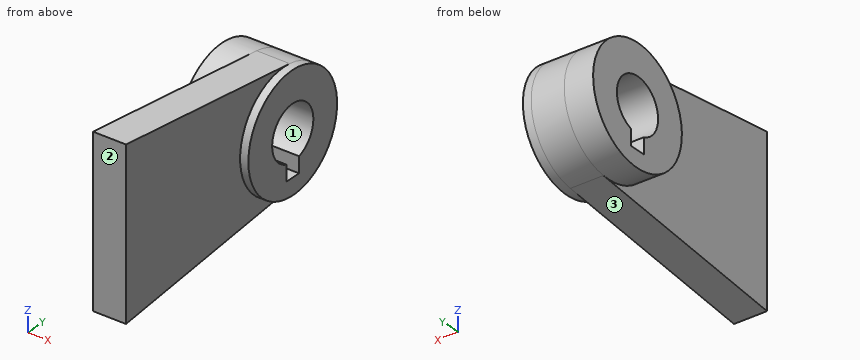
from build123d import *
from build123d.topology import SkipClean

# Parameters (mm, degrees)
SALIENTE_EXTRUIR3_DEPTH = 16
CROQUIS6_R              = 28
SALIENTE_EXTRUIR4_DEPTH = 4
SALIENTE_EXTRUIR5_START = 14
CROQUIS7_R              = 28
SALIENTE_EXTRUIR5_DEPTH = 14
CORTAR_EXTRUIR1_DEPTH   = 106.924501415


with BuildPart() as part:
    # Croquis5 → Saliente-Extruir3 (new body)
    with BuildSketch(Plane(origin=(0, 0, 0), x_dir=(0, 0, -1), z_dir=(1, 0, 0))):
        with BuildLine():
            Line((40, -36), (27.806896216, 67.282758707))
            ThreePointArc((27.806896216, 67.282758707), (-4.12e-07, 92), (-27.806896887, 67.282758534))
            Line((-27.806896887, 67.282758534), (-40, -36))
            Line((-40, -36), (40, -36))
        make_face()
    extrude(amount=SALIENTE_EXTRUIR3_DEPTH)

    # Croquis6 → Saliente-Extruir4 (add)
    with BuildSketch(Plane(origin=(16, 0, 0), x_dir=(0, 0, -1), z_dir=(1, 0, 0))):
        with Locations(Location((-3.25e-07, 64, 0), (0, 0, 173.267078851))):
            Circle(CROQUIS6_R)
    extrude(amount=SALIENTE_EXTRUIR4_DEPTH)

    # Croquis7 → Saliente-Extruir5 (add)
    with SkipClean():  # the faces are left unmerged after this step: merging them gives an invalid solid
        with BuildSketch(Plane.ZY.offset(SALIENTE_EXTRUIR5_START)):
            with Locations((3.25e-07, 64)):
                Circle(CROQUIS7_R)
        extrude(amount=-SALIENTE_EXTRUIR5_DEPTH)

    # Croquis8 → Cortar-Extruir1 (cut, through all)
    with SkipClean():  # the faces are left unmerged after this step: merging them gives an invalid solid
        with BuildSketch(Plane(origin=(20, 0, 0), x_dir=(0, 0, -1), z_dir=(1, 0, 0))):
            with BuildLine():
                Line((19.999999675, 68), (19.999999675, 60))
                Line((19.999999675, 60), (12.369316552, 60))
                ThreePointArc((12.369316552, 60), (-13.000000325, 64), (12.369316552, 68))
                Line((12.369316552, 68), (19.999999675, 68))
            make_face()
        extrude(amount=-CORTAR_EXTRUIR1_DEPTH, mode=Mode.SUBTRACT)


solid = part.part
Input: part model. Units: mm. Frame: model coordinates. Face numbers are marked on the shaded views. Coordinates: 2 decimals unless noted, no trailing zeros. Loops run counter-clockwise (first coordinate to the right, second up) from the corner with the lowest first, then second, coordinate; pieces in that order, holes last.
(1) First-contact query: pin 1 Ø3 at (x, z) = (1.5, 23) entering from +Y; pin 2 Ø4 at (x, z) = (-10.5, 11.5) entering from -Y; pin 3 Ø5 at (y, z) = (-14, 0) entering from +X. Flat tips, straight axial feed; report the tip coordinate or a pass-through.
(2) Section C-C on y = 64. Return the cut outline in (x, z).
(3) Section B-B on x = 11. Return the cut outline in (y, z).
(4) Section A-A on z = 0. Return the cut outline in (x, y), then the cut area to 3 significant figures.
(5) Section D-D on z = -15. Return the cut outline in (x, y), then the cut area to 3 significant figures.
(6) Pull-direction query (Z, two-part tool) for the marked faces 1, 2 and 3; classes: released by +Z, released by -Z, zero draft, split by the parting line, or undercut.
(7) Material intervals for probe 1 along Z at (x, y) = (-6.5, 64); probe 2 along Y at (x, z) = (-4, 0); probe 3 along X at (y, z) = (-11, 31), sorted ascending.
Data:
1. pin 1: stops at y = 81.94
1. pin 2: stops at y = 37.66
1. pin 3: stops at x = 16
2. outline: (-14, -28) - (0, -28) - (0, -28.19) - (16, -28.19) - (16, -28) - (20, -28) - (20, -20) - (-14, -20) - close; (-14, 13) - (20, 13) - (20, 28) - (16, 28) - (16, 28.19) - (0, 28.19) - (0, 28) - (-14, 28) - close
3. outline: (-36, -40) - (67.28, -27.81) arc R28 ccw to (67.28, 27.81) - (-36, 40) - close; hole (60, -20) - (68, -20) - (68, -12.37) arc R13 ccw (long way) to (60, -12.37) - close
4. outline: (-14, 36) - (0, 36) - (0, -36) - (16, -36) - (16, 36) - (20, 36) - (20, 51) - (-14, 51) - close; (-14, 77) - (20, 77) - (20, 92) - (-14, 92) - close
4. area: 2,170 mm2
5. outline: (-14, 40.36) - (0, 40.36) - (0, -36) - (16, -36) - (16, 40.36) - (20, 40.36) - (20, 60) - (-14, 60) - close; (-14, 68) - (20, 68) - (20, 87.64) - (-14, 87.64) - close
5. area: 2,560 mm2
6. face 1: undercut
6. face 2: zero draft
6. face 3: released by -Z
7. probe 1: z = -28 to -20, 13 to 28
7. probe 2: y = 36 to 51, 77 to 92
7. probe 3: x = 0 to 16
